```python
from build123d import *

# Parameters (mm, degrees)
SKETCH_1_W      = 27.5
SKETCH_1_H      = 13.5
EXTRUDE_1_DEPTH = 2.5
SKETCH_2_W      = 2.5
SKETCH_2_H      = 13.5
EXTRUDE_2_DEPTH = 3
SKETCH_5_R      = 0.25
EXTRUDE_6_DEPTH = 3
SKETCH_6_R      = 2.5
EXTRUDE_7_DEPTH = 20


with BuildPart() as part:
    # Эскиз1 → Бобышка-Вытянуть1 (new body)
    with BuildSketch(Plane(origin=(0, 0, 0), x_dir=(1, 0, 0), z_dir=(0, 1, 0))):
        Rectangle(SKETCH_1_W, SKETCH_1_H)
    extrude(amount=EXTRUDE_1_DEPTH)

    # Эскиз2 → Бобышка-Вытянуть2 (add)
    with BuildSketch(Plane.XZ):
        with Locations((12.5, 0)):
            Rectangle(SKETCH_2_W, SKETCH_2_H)
    extrude(amount=-EXTRUDE_2_DEPTH)

    # Эскиз5 → Бобышка-Вытянуть6 (add)
    with BuildSketch(Plane(origin=(0, 2.5, 0), x_dir=(1, 0, 0), z_dir=(0, 1, 0))):
        with Locations(Location((-12.75, -1.5, 0), (0, 0, 90))):
            Circle(SKETCH_5_R)
    extrude(amount=EXTRUDE_6_DEPTH)

    # Эскиз6 → Бобышка-Вытянуть7 (add)
    with BuildSketch(Plane(origin=(0, 5.5, 0), x_dir=(1, 0, 0), z_dir=(0, 1, 0))):
        with Locations(Location((-10.5, -1.5, 0), (0, 0, 180))):
            Circle(SKETCH_6_R)
    extrude(amount=EXTRUDE_7_DEPTH)


solid = part.part
```
Source: CAD feature listing. Evaluate the final solid. Frame: model axes, mm. Give positions to 0.01 mm unless a question says otherwise; leave off trailing zeros. Order: outer loops, then holes, each group sorted by start corner. A loop starts at its lowest first (then second) coordinate and runs counter-clockwise, first axis right, second up.
(1) Pull-direction query (Y, two-part tool) for faces 1 (the face through (-8, 15.4, 1.6)), 2 (the face through (12, 3, 0)), 3 (the face through (-10, 5.5, 2)); classes: +Y half, -Y half, draft (parallel to the pull), parting line (faces both ways), or undercut.
(2) Section query D-D (x = -1). Return the cut outline in (y, z).
(3) Section query B-B (z = -0.5). Return the cut outline in (x, y), plus the area to 3 significant figures.
(4) Material intervals for line 1 along Y through (x, z) = (-9.5, 2); line 2 along Y through (x, z) = (8.5, -1); line 3 along Y through (x, z) = (11.75, 1), sorted ascending.
(5) Contact query for flat-ended pins moving along their axis: P1, Ø4, axis at y = 5.5, z = 1.5, coming from the -X side; P2, Ø1.2, axis at x = 13, z = 0, coming from the +Y side. Output: stop coordinate, or through.
(6) Section query C-C (y = 14). Return the cut outline in (x, z).
(7) Section query A-A (x = -10.5). Return the cut outline in (y, z), plus the area to 3 significant figures.
Outcome:
1. face 1: draft
1. face 2: +Y half
1. face 3: undercut
2. outline: (0, -6.75) - (2.5, -6.75) - (2.5, 6.75) - (0, 6.75) - close
3. outline: (-13.75, 0) - (13.75, 0) - (13.75, 3) - (11.25, 3) - (11.25, 2.5) - (-13.75, 2.5) - close; (-12, 5.5) - (-9, 5.5) - (-9, 25.5) - (-12, 25.5) - close
3. area: 130 mm2
4. line 1: y = 0 to 2.5, 5.5 to 25.5
4. line 2: y = 0 to 2.5
4. line 3: y = 0 to 3
5. P1: stops at x = -13
5. P2: stops at y = 3
6. outline: circle Ø5 at (-10.5, 1.5)
7. outline: (0, -6.75) - (2.5, -6.75) - (2.5, 6.75) - (0, 6.75) - close; (5.5, -1) - (25.5, -1) - (25.5, 4) - (5.5, 4) - close
7. area: 134 mm2
